The listing builds one solid part. Answer for the finished solid, in the listing's coordinates (mm). A direction names the side the tool comes from. Coordinates: 2 decimals unless noted, no trailing zeros. Write each loop counter-clockwise with the first axis right and the second up, starting at its lowest first coordinate (ties: lowest second). Pieces come first, ordered by that corner, then holes.
from build123d import *

# Parameters (mm, degrees)
F0_W     = 80
F0_H     = 60
F1_DEPTH = 50
F3_DEPTH = 25
F4_R     = 10
F5_DEPTH = 25
F6_R     = 10
F7_DEPTH = 15


with BuildPart() as f1:
    # F0 (on Top) → F1 (new body)
    with BuildSketch(Plane.XY):
        Rectangle(F0_W, F0_H)
    extrude(amount=F1_DEPTH)

    # F2 (on face) → F3 (join)
    with BuildSketch(Plane.XY.offset(50)):
        with BuildLine():
            ThreePointArc((-40, 0), (-30, -10), (-20, 0))
            ThreePointArc((-20, 0), (-30, 10), (-40, 0))
        make_face()
    extrude(amount=F3_DEPTH)

    # F4 (on face) → F5 (join)
    with BuildSketch(Plane.XY.offset(50)):
        Circle(F4_R)
    extrude(amount=F5_DEPTH)

    # F6 (on face) → F7 (cut)
    with BuildSketch(Plane.XZ.offset(30)):
        with Locations((0, 15)):
            Circle(F6_R)
    extrude(amount=-F7_DEPTH, mode=Mode.SUBTRACT)


solid = f1.part
1. A tool of negligible diameter and unlimited length cuts with its end or side. For faces 4 (the flat face through (-30, 0, 75)), 5 (the cylindrical face through (-1.302, -22.605, 24.915)), 6 (the cylindrical face through (-40, 0, 62)), from which of +Z, -Z, +X, -X, +Y, -Y can it reach the whole face along a straight path? Write none if from no direction.
Results found:
face 4: +Z, +X, -X, +Y, -Y
face 5: -Y
face 6: +Z
2. Section B-B on y = 6 is taken. Give the vertices of the cut face in (x, z).
Results found:
outline: (-40, 0) - (40, 0) - (40, 50) - (8, 50) - (8, 75) - (-8, 75) - (-8, 50) - (-22, 50) - (-22, 75) - (-38, 75) - (-38, 50) - (-40, 50) - close
3. For a pull along Z with two mould halves and no side action, classify faces 1 (the flat face through (0, -15, 15)), 2 (the flat face through (-1, 30, 25)), 3 (the flat face through (0, 0, 75)) as pulls with the +Z half, pulls with the -Z half, needs draft (parallel to the pull), parting line crosses it, or undercut.
Results found:
face 1: undercut
face 2: needs draft
face 3: pulls with the +Z half
4. Section C-C on z = 55 is taken. Give the vertices of the cut face in (x, y).
Results found:
outline: circle Ø20 at (-30, 0); circle Ø20 at (0, 0)
5. Flat-ended cylindrical pins translate along their axes: P1, Ø6, axis at x = -29.5, y = -12, coming from the +Z side; P2, Ø6, axis at x = -29.5, z = 60, coming from the +Y side; P3, Ø10, axis at x = -4.5, z = 14, coming from the -Y side. Find the tip coordinate at first contact, or state that the pin passes through.
Results found:
P1: stops at z = 75
P2: stops at y = 10
P3: stops at y = -15
6. Find the intervals of material crossed by L1, parallel to Z at x = 0, y = -26; L2, parallel to Z at x = 6, y = 8.5; L3, parallel to X at y = -2.5, z = 53, in increasing order.
Results found:
L1: z = 0 to 5, 25 to 50
L2: z = 0 to 50
L3: x = -39.68 to -20.32, -9.68 to 9.68
7. Section A-A on x = -30 is taken. Give the vertices of the cut face in (y, z).
Results found:
outline: (-30, 0) - (30, 0) - (30, 50) - (10, 50) - (10, 75) - (-10, 75) - (-10, 50) - (-30, 50) - close
8. Section D-D on z = 15 is taken. Give the vertices of the cut face in (x, y).
Results found:
outline: (-40, -30) - (-10, -30) - (-10, -15) - (10, -15) - (10, -30) - (40, -30) - (40, 30) - (-40, 30) - close
